from build123d import *

# Parameters (mm, degrees)
SKETCH2_R          = 2
CUT_EXTRUDE1_DEPTH = 10


with BuildPart() as part:
    # Sketch1 → Revolve1 (revolve)
    with BuildSketch(Plane.XY, mode=Mode.PRIVATE) as revolve1_sk:
        with BuildLine():
            Line((13.5, 0), (19.5, 0))
            Line((19.5, 0), (19.5, 8))
            Line((19.5, 8), (18, 8))
            Line((18, 8), (18, 9.5))
            Line((18, 9.5), (24.5, 9.5))
            Line((24.5, 9.5), (24.5, 20))
            Line((24.5, 20), (20.5, 23))
            Line((20.5, 23), (17, 23))
            ThreePointArc((17, 23), (16.292893219, 23.292893219), (16, 24))
            Line((16, 24), (16, 59.5))
            ThreePointArc((16, 59.5), (16.292893219, 60.207106781), (17, 60.5))
            Line((17, 60.5), (26.5, 60.5))
            Line((26.5, 60.5), (26.5, 65.5))
            Line((26.5, 65.5), (9.5, 65.5))
            Line((9.5, 65.5), (9.5, 48))
            Line((9.5, 48), (6.5, 44.5))
            Line((6.5, 44.5), (6.5, 37.5))
            Line((6.5, 37.5), (7, 37))
            Line((7, 37), (7, 17))
            Line((7, 17), (6.5, 16.5))
            Line((6.5, 16.5), (6.5, 8))
            Line((6.5, 8), (13.5, 8))
            Line((13.5, 8), (13.5, 0))
        make_face()
    revolve(revolve1_sk.sketch.rotate(Axis((0, 0, 0), (0, 1, 0)), 90), axis=Axis((0, 0, 0), (0, 1, 0)))

    # Sketch2 → Cut-Extrude1 (cut)
    with BuildSketch(Plane(origin=(0, 65.5, 0), x_dir=(1, 0, 0), z_dir=(0, 1, 0))):
        with Locations(Location((21.5, 0, 0), (0, 0, 270))):
            Circle(SKETCH2_R)
        with Locations(Location((-21.5, 0, 0), (0, 0, 270))):
            Circle(SKETCH2_R)
    extrude(amount=-CUT_EXTRUDE1_DEPTH, mode=Mode.SUBTRACT)


solid = part.part
Here's how the part is built. I have some questions about the finished solid (model axes, mm). A direction names the side the tool comes from. Round coordinates to 2 decimals unless told otherwise and drop trailing zeros. Order: outer loops, then holes, each group sorted by start corner. A loop starts at its lowest first (then second) coordinate and runs counter-clockwise, first axis right, second up. Notation, with made-up numbers: M 49,-27 L 59,-27 A25 ccw 59,-10 Z; hole C -38,20 d8. An arc over 180 degrees is marked long. One line per question, with ' | ' between items.
1) We'd pull the mould along Y, two halves only. Please class faces 6 (the cylindrical face through (15.62, 42, 3.47)), 7 (the flat face through (-3, 8, 6)), 8 (the flat face through (-0.4, 60.5, 17.3)), 9 (the cylindrical face through (-19.517, 63.035, -0.26)): released by +Y, released by -Y, zero draft, split by the parting line, or undercut.
Checked values:
face 6: undercut | face 7: released by -Y | face 8: undercut | face 9: zero draft
2) I'm going to push flat-ended pins straight in: pin 1 Ø5 at (y, z) = (47.5, -2) entering from +X; pin 2 Ø1.5 at (x, y) = (-4.5, 25) entering from -Z; pin 3 Ø10 at (x, z) = (4, -1) entering from +Y. Where does each tip first touch, or does it pass through?
Checked values:
pin 1: stops at x = 16 | pin 2: stops at z = -15.55 | pin 3: stops at y = 47.56
3) Imagine slicing it at D-D, the plane y = 51. Write out the boundary of the cut face in (x, z), plus the area to 3 significant figures.
Checked values:
outline: C 0,0 d32; hole C 0,0 d19 | area: 521 mm²
4) I need wall thicknesses on line 1 (X direction, y = 62.85, z = 0); line 2 (Y direction, x = 3, z = 18); line 3 (X direction, y = 43, z = 0). Which ranges of each line are inside material? Lowest first, please.
Checked values:
line 1: x = -26.5 to -23.5, -19.5 to -9.5, 9.5 to 19.5, 23.5 to 26.5 | line 2: y = 0 to 8, 9.5 to 23, 60.5 to 65.5 | line 3: x = -16 to -6.5, 6.5 to 16
5) Imagine slicing it at A-A, the plane y = 40.5. Write out the boundary of the cut face in (x, z).
Checked values:
outline: C 0,0 d32; hole C 0,0 d13
6) Imagine slicing it at B-B, the plane z = 0. Count the separate pieces of the cut face and the enclosed holes in it, plus the area to 3 significant figures.
Checked values:
separate pieces: 4 | enclosed holes: 0 | area: 1,340 mm²
7) On a 3-axis mill with a long thin cutter (end or side, diameter ignored), from which of +Z, -Z, +X, -X, +Y, -Y can I reach the whole of each face in a straight line? I mean faces 1 (the flat face through (0, 65.5, -11)), 2 (the cylindrical face through (-12.165, 8.76, 13.267)), 3 (the cylindrical face through (3.955, 12.19, 5.158)), 4 (the cylindrical face through (-19.334, 4.056, 2.539)), 5 (the cylindrical face through (23.483, 63.035, -0.26)). Say none if no direction works.
Checked values:
face 1: +Z, -Z, +X, -X, +Y | face 2: none | face 3: +Y, -Y | face 4: -Y | face 5: +Y
